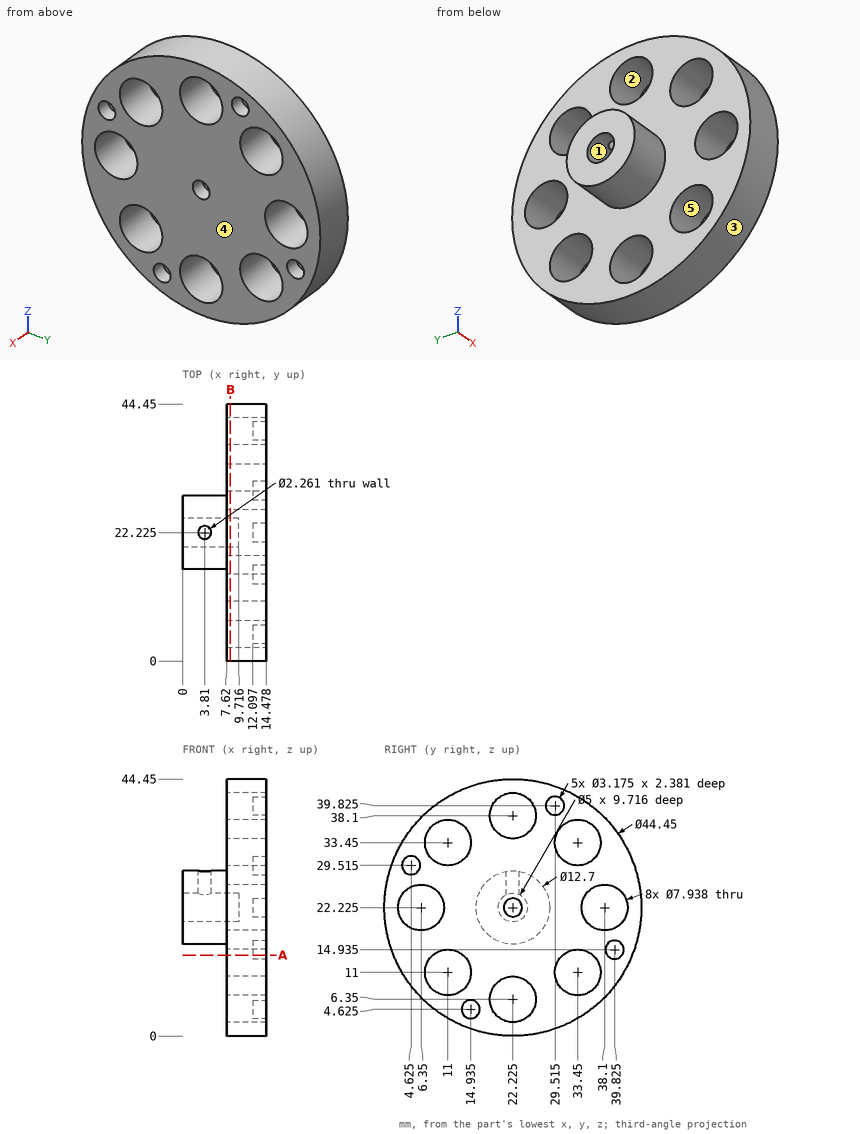
For this review, use the dimensioned drawing (mm, ordinates from the lowest corner) and the shaded views. A direction names the side the tool comes from. Give positions to 0.01 mm unless a question says otherwise; leave off trailing zeros. Order: outer loops, then holes, each group sorted by start corner. A loop starts at its lowest first (then second) coordinate and runs counter-clockwise, first axis right, second up. Notation, with made-up numbers: (58, 43.5) - (96, 43.5) arc R19 cw to (96, 57.5) - close; hole circle Ø7 at (13.5, 2.5). An arc over 180 degrees is marked (long way). Use a Markdown table: item, result. Add a question column.
(1) Add section A-A on z = 14. Give the boundary of the cut face in (x, y), then the cut area to 3 significant figures.
(2) Add section B-B on x = 8.25. Give the number of separate pieces and of enclosed holes in the cut face, then the cut area to 3 significant figures.
(3) Mouldability with a two-part tool opening along Z and no side actions: class the marked faces 3, 4 and 5 as +Z half, -Z half, draft (parallel to the pull), parting line (faces both ways), or undercut.
(4) Clearance check with flat-ended pins moving along their axes: P1, Ø1.6, axis at y = 5, z = 29, coming from the +X side; P2, Ø5, axis at y = 38.1, z = 22.225, coming from the -X side; P3, Ø4, axis at x = 3, z = 16, coming from the +Y side (1 decimal); P4, Ø2.5, axis at y = 21.5, z = 23, coming from the -X side (1 decimal). State where each tip first meets the part, or that it passes through.
(5) Wall thickness on probe 1 along Y at (x, z) = (9.5, 22.5); probe 2 along X at (y, z) = (2, 16.5); probe 3 along X at (y, z) = (21.5, 21.5) (1 decimal): over which ranges is each line inside the solid? List them lowest first. Write a range as [from, to].
(6) Machinability: for the marked faces 1 and 2, which of the approach directions +Z, -Z, +X, -X, +Y, -Y give a long, thin tool a straight path to every point of the face, cutting with its end or side? Answer none if there is none.
Report:
| question | item | result |
|---|---|---|
| 1 | outline | (7.62, 1.58) - (14.48, 1.58) - (14.48, 8.4) - (7.62, 8.4) - close; (7.62, 13.6) - (14.48, 13.6) - (14.48, 30.85) - (7.62, 30.85) - close; (7.62, 36.05) - (14.48, 36.05) - (14.48, 38.54) - (12.1, 38.54) - (12.1, 41.11) - (14.48, 41.11) - (14.48, 42.87) - (7.62, 42.87) - close |
| 1 | area | 206 mm² |
| 2 | separate pieces | 1 |
| 2 | enclosed holes | 9 |
| 2 | area | 1,140 mm² |
| 3 | face 3 | parting line |
| 3 | face 4 | draft |
| 3 | face 5 | undercut |
| 4 | P1 | stops at x = 12.1 |
| 4 | P2 | passes through |
| 4 | P3 | stops at y = 27 |
| 4 | P4 | stops at x = 9.7 |
| 5 | probe 1 | y = [0, 2.39], [10.31, 19.74], [24.71, 34.14], [42.06, 44.45] |
| 5 | probe 2 | x = [7.62, 14.48] |
| 5 | probe 3 | x = [9.7, 12.1] |
| 6 | face 1 | -X |
| 6 | face 2 | +X, -X |
